Work out the finished part from the listing and answer in its coordinate system (mm). A direction names the side the tool comes from. Round coordinates to 2 decimals unless told otherwise and drop trailing zeros. Order: outer loops, then holes, each group sorted by start corner. A loop starts at its lowest first (then second) coordinate and runs counter-clockwise, first axis right, second up. Notation, with made-up numbers: M -20,64.5 L 24,64.5 A23 ccw 24,81.5 Z; hole C 83,28.25 d1. An arc over 180 degrees is marked long. Return JSON: item names as keys, results as strings.
from build123d import *

# Parameters (mm, degrees)
SKETCH1_R          = 31.623
EXTRUDE1_DEPTH     = 91.948
CHAMFER1_SIZE      = 0.762
SKETCH6_R          = 22.225
EXTRUDE2_DEPTH     = 5.969
SKETCH7_W          = 35.56
SKETCH7_H          = 14.2875
CUT_EXTRUDE4_DEPTH = 19.84248
HOLE1_D            = 4.7498
HOLE1_DEPTH        = 4.7498
CIRPATTERN1_COUNT  = 4
LPATTERN2_COUNT    = 2
LPATTERN2_PITCH    = 31.75


with BuildPart() as part:
    # Sketch1 → Extrude1 (new body)
    with BuildSketch(Plane.XY):
        Circle(SKETCH1_R)
    extrude(amount=EXTRUDE1_DEPTH)

    # Sketch2 → Cut-Revolve1 (revolve, cut)
    with BuildSketch(Plane(origin=(0, 0, 0), x_dir=(1, 0, 0), z_dir=(0, 1, 0)), mode=Mode.PRIVATE) as cut_revolve1_sk:
        Polygon((31.623, -91.948), (31.623, -77.978), (30.353, -79.248), (30.353, -91.948), align=None)
    revolve(cut_revolve1_sk.sketch.rotate(Axis((0, 0, 0), (0, 0, 1)), 180), axis=Axis((0, 0, 0), (0, 0, 1)), mode=Mode.SUBTRACT)  # turned: the seam where the file's is

    # Sketch3 → Cut-Revolve2 (revolve, cut)
    with BuildSketch(Plane(origin=(0, 0, 0), x_dir=(1, 0, 0), z_dir=(0, 1, 0)), mode=Mode.PRIVATE) as cut_revolve2_sk:
        Polygon((30.353, 0), (30.353, -1.524), (31.623, -2.794), (31.623, 0), align=None)
    revolve(cut_revolve2_sk.sketch.rotate(Axis((0, 0, 0), (0, 0, -1)), 180), axis=Axis((0, 0, 0), (0, 0, -1)), mode=Mode.SUBTRACT)  # turned: the seam where the file's is

    # S2D0002 → Cut-Revolve3 (revolve, cut)
    with BuildSketch(Plane(origin=(0, 0, 0), x_dir=(0, -1, 0), z_dir=(1, 0, 0)), mode=Mode.PRIVATE) as cut_revolve3_sk:
        Polygon((-4.9403, -91.694), (-1.6002, -91.694), (-1.6002, -91.948), (-11.1252, -91.948), (-11.1252, -77.724), (-6.1468, -77.724), (-6.1468, -88.477393135), (-5.482893135, -89.1413), align=None)
    cut_revolve3 = revolve(cut_revolve3_sk.sketch.rotate(Axis((0, 11.1252, 14.6685), (0, 0, -1)), 270), axis=Axis((0, 11.1252, 14.6685), (0, 0, -1)), mode=Mode.SUBTRACT)  # turned: the seam where the file's is

    # Chamfer1
    chamfer1_edges = [part.edges().sort_by_distance(p)[0] for p in [
        (30.353, 0, 91.948),
    ]]
    chamfer(chamfer1_edges, length=CHAMFER1_SIZE)

    # Sketch6 → Extrude2 (add)
    with BuildSketch(Plane(origin=(0, 0, 0), x_dir=(-1, 0, 0), z_dir=(0, 0, -1))):
        with Locations(Location((0, 0, 0), (0, 0, 180))):  # turned: the seam where the file's is
            Circle(SKETCH6_R)
    extrude(amount=EXTRUDE2_DEPTH)

    # Sketch7 → Revolve1 (revolve)
    with BuildSketch(Plane(origin=(0, 0, 0), x_dir=(0, 0, -1), z_dir=(1, 0, 0)), mode=Mode.PRIVATE) as revolve1_sk:
        with Locations((23.749, -7.14375)):
            Rectangle(SKETCH7_W, SKETCH7_H)
    revolve(revolve1_sk.sketch.rotate(Axis((0, 0, 0), (0, 0, -1)), 270), axis=Axis((0, 0, 0), (0, 0, -1)))  # turned: the seam where the file's is

    # S2D0001 → Cut-Revolve5 (revolve, cut)
    with BuildSketch(Plane(origin=(0, 0, 0), x_dir=(1, 0, 0), z_dir=(0, 1, 0))):
        Polygon((5.5499, 39.461277746), (5.5499, 25.146), (0, 25.146), (0, 41.529), (6.7437, 41.529), align=None)
    revolve(axis=Axis((0, 0, 31.308359971), (0, 0, -1)), mode=Mode.SUBTRACT)

    # Sketch9 → Cut-Revolve6 (revolve, cut)
    with BuildSketch(Plane(origin=(0, 0, 0), x_dir=(0, -1, 0), z_dir=(1, 0, 0)), mode=Mode.PRIVATE) as cut_revolve6_sk:
        with BuildLine():
            Line((-14.2875, 31.623), (-14.097, 32.385))
            Line((-14.097, 32.385), (-14.097, 40.513))
            ThreePointArc((-14.097, 40.513), (-13.996678675, 41.056796865), (-13.708922533, 41.529))
            Line((-13.708922533, 41.529), (-14.2875, 41.529))
            Line((-14.2875, 41.529), (-14.2875, 31.623))
        make_face()
    revolve(cut_revolve6_sk.sketch.rotate(Axis((0, 0, -12.65936), (0, 0, -1)), 90), axis=Axis((0, 0, -12.65936), (0, 0, -1)), mode=Mode.SUBTRACT)  # turned: the seam where the file's is

    # Sketch13 → Cut-Extrude4 (cut, symmetric)
    with BuildSketch(Plane(origin=(0, 0, 0), x_dir=(1, 0, 0), z_dir=(0, 1, 0))):
        Polygon((12.573, 41.529), (12.573, 33.9598), (14.2875, 32.2453), (14.2875, 41.529), align=None)
        Polygon((-12.573, 41.529), (-12.573, 33.9598), (-14.2875, 32.2453), (-14.2875, 41.529), align=None)
    extrude(amount=CUT_EXTRUDE4_DEPTH, both=True, mode=Mode.SUBTRACT)

    # Hole1
    with Locations(Plane(origin=(-21.462812129, 21.462812129, 85.598), x_dir=(0.707106781, 0.707106781, 0), z_dir=(-0.707106781, 0.707106781, 0))):
        with Locations((0, 0)):
            hole1 = Hole(HOLE1_D / 2, depth=HOLE1_DEPTH)

    # CirPattern1: Hole1 ×4 about axis
    cirpattern1_axis = Axis((0, 0, 0), (0, 0, 1))
    for i in range(1, CIRPATTERN1_COUNT):
        add(hole1.rotate(cirpattern1_axis, i * 360 / CIRPATTERN1_COUNT), mode=Mode.SUBTRACT)

    # LPattern2: Cut-Revolve3 ×2
    with Locations(*[(0, -i * LPATTERN2_PITCH, 0) for i in range(1, LPATTERN2_COUNT)]):
        add(cut_revolve3, mode=Mode.SUBTRACT)


solid = part.part
Item 1: Find section B-B (z = 71). Determine the outline of the cut face in (x, y), plus the area to 3 significant figures.
Output:
{"outline": "C 0,0 d63.25", "area": "3,140 mm^2"}
Item 2: The mould has two halves that part along Y. Classify faces 5 (the flat face through (-3, -6.3, -41.529)), 6 (the cylindrical face through (-16.4, -15, -2.9)), 7 (the flat face through (-18.08, 18.13, 85.56)), 8 (the flat face through (-6.2, 13.1, 91.694)): pulls with the +Y half, pulls with the -Y half, needs draft (parallel to the pull), parting line crosses it, or undercut.
Output:
{"face 5": "needs draft", "face 6": "parting line crosses it", "face 7": "undercut", "face 8": "undercut"}
Item 3: Find section A-A (z = -13). Determine the outline of the cut face in (x, y) (1 decimal), plus the area to 3 significant figures.
Output:
{"outline": "C 0,0 d28.6", "area": "641 mm^2"}
Item 4: Consider line 1 along Y through (x, z) = (0, 84); line 2 along Z through (x, y) = (21, -15); line 3 along Z through (x, y) = (-9, 10). Determine where each line is inside the solid, lowest interval first. Write a range as [from, to].
Output:
{"line 1": "y = [-30.35, -25.6], [-15.65, 6.15], [16.1, 30.35]", "line 2": "z = [0, 91.95]", "line 3": "z = [-41.53, 91.69]"}
Item 5: Which of the six approach directions +Z, -Z, +X, -X, +Y, -Y give full straight-line access (tool end or side, diameter ignored) to faces 1 (the cylindrical face through (-28.95, 9.12, 0.77)), 2 (the flat face through (-12.573, 0, -38)), 3 (the flat face through (18.08, -18.13, 85.56)), 4 (the flat face through (0, -27, 91.694))?
Output:
{"face 1": "-Z", "face 2": "-Z, -X, +Y, -Y", "face 3": "none", "face 4": "+Z"}
Item 6: Each of these flat-tipped pins is pushed along its axis until it touches: pin 1 (5.5 mm diameter, centred on x = -0.5, y = 0, fed in from -Z); pin 2 (9.5 mm diameter, centred on x = 3.5, y = -24, fed in from +Z); pin 3 (8 mm diameter, centred on x = 0, y = -21.5, fed in from +Z); pin 4 (4 mm diameter, centred on y = -12.5, z = 14, fed in from -X). Where does it stop, or does it pass through?
Output:
{"pin 1": "stops at z = -25.15", "pin 2": "stops at z = 91.95", "pin 3": "stops at z = 77.72", "pin 4": "stops at x = -29.83"}
